Read the model definition and answer for the solid it produces. Units are mm, in the model's axes. A direction names the side the tool comes from. Coordinates: 2 decimals unless noted, no trailing zeros. Write each loop counter-clockwise with the first axis right and the second up, starting at its lowest first coordinate (ties: lowest second). Pieces come first, ordered by that corner, then holes. Notation, with made-up numbers: (80.25, 88.5) -> (138.25, 88.5) arc R19 cw to (138.25, 100.5) -> close; hole circle Ø6 at (42, -27.5). An arc over 180 degrees is marked (long way). Answer as a JSON object with one key per item and string values. Group by question number.
(1) Find section A-A (z = 7.25). Give the vertices of the cut face in (x, y).
(2) Flat-ended cylindrical pins translate along their axes: P1, Ø1.5, axis at x = 4.5, y = 18.5, coming from the -Z side; P2, Ø5.5, axis at y = 10.5, z = 5, coming from the +X side; P3, Ø4, axis at x = 11.5, z = 10, coming from the -Y side. Find the tip coordinate at first contact, or state that the pin passes through.
(3) Find section D-D (y = 5.5). Give the vertices of the cut face in (x, z), then the cut area to 3 significant figures.
(4) Find section B-B (x = 4.1). Give the vertices of the cut face in (y, z).
(5) Straight lines are drawn through the part: L1, parallel to Y at x = 4.1, z = 10.6; L2, parallel to X at y = 19, z = 2.75; L3, parallel to Y at x = 3.5, z = 5.5. For each, find the intervals that lie inside material, in ascending order.
(6) Find section C-C (y = 15.24). Give the vertices of the cut face in (x, z) (3 decimals).
(7) Which of the six approach directions +Z, -Z, +X, -X, +Y, -Y give full straight-line access (tool end or side, diameter ignored) to faces 4 (the face through (6.2, 15.5, 0.8)), 5 (the face through (4, 28.88, 7)), 6 (the face through (10.85, 15.27, 10.61))?
(8) For a pull along Y with two mould halves and no side action, classify faces 1 (the face through (14.034, 15.081, 10.611)), 2 (the face through (10, 15, 9.8)), 3 (the face through (1.6, 15, 5)) as +Y half, -Y half, draft (parallel to the pull), parting line (faces both ways), or undercut.
Autodesk Inventor part; units mm, degrees
ref_plane "YZ Plane" through (0, 0, 0) normal (1, 0, 0) x (0, 1, 0)
ref_plane "XZ Plane" through (0, 0, 0) normal (0, 1, 0) x (-1, 0, 0)
ref_plane "XY Plane" through (0, 0, 0) normal (0, 0, 1) x (1, 0, 0)
sketch "Sketch1" plane through (0, 0, 0) normal (0, 0, 1) x (1, 0, 0)
  line L0 (0, 0) -> (8.2, 0)
  line L1 (8.2, 0) -> (8.2, 30.48)
  line L2 (8.2, 30.48) -> (0, 30.48)
  line L3 (0, 30.48) -> (0, 0)
  line L4 (6.6, 28.88) -> (6.6, 1.6)
  line L5 (6.6, 1.6) -> (1.6, 1.6)
  line L6 (1.6, 1.6) -> (1.6, 28.88)
  line L7 (1.6, 28.88) -> (6.6, 28.88)
  dimension "d0" = 30.48
  dimension "d1" = 8.2
  dimension "d2" = 1.6
extrude "Extrusion1" add sketch "Sketch1" along normal blind 11.4
sketch "Sketch2" plane through (0, 0, 0) normal (0, -1, 0) x (1, 0, 0)
  line L0 (6.6, 0) -> (6.6, 11.4)
  line L1 (1.6, 0) -> (1.6, 11.4)
  line L2 (0, 0) -> (8.2, 0)
  line L3 (1.6, 0) -> (1.6, 2.4)
  line L4 (1.6, 0) -> (1.6, 11.4)
  line L5 (6.6, 0) -> (6.6, 2.4)
  line L6 (6.6, 0) -> (6.6, 11.4)
  line L7 (1.6, 0) -> (6.6, 0)
  arc A0 (6.6, 2.4) -> (1.6, 2.4) centre (4.1, 2.4) ccw
  dimension "d5" = 2.4
  dimension "d6" = 2.4
extrude "Extrusion2" cut sketch "Sketch2" against normal up to surface (30.48 mm away)
sketch "Sketch3" plane through (0, 0, 0) normal (-1, 0, 0) x (0, 0, 1)
  line L0 (0, 30.48) -> (0, 0)
  line L1 (0, 0) -> (11.4, 0)
  line L2 (11.4, 30.48) -> (11.4, 0)
  line L3 (0, 30.48) -> (11.4, 30.48)
  line L4 (0, 0) -> (11.4, 0)
  line L5 (11.4, 30.48) -> (9.8, 30.48)
  line L6 (9.8, 30.48) -> (9.8, 0)
  line L7 (9.8, 0) -> (11.4, 0)
  line L8 (11.4, 0) -> (11.4, 30.48)
  dimension "d9" = 1.6
extrude "Extrusion3" add sketch "Sketch3" against normal up to next contours L3 L2 L1 L6
sketch "Sketch4" plane through (0, 0, 11.4) normal (0, 0, 1) x (1, 0, 0)
  line L0 (0, 0) -> (8.2, 0)
  line L1 (8.2, 0) -> (8.2, 30.48)
  line L2 (8.2, 30.48) -> (0, 30.48)
  line L3 (0, 30.48) -> (0, 0)
  line L4 (6.6, 0) -> (1.6, 0)
  line L5 (4.1, 0) -> (4.1, 30.48)
  line L6 (1.6, 30.48) -> (6.6, 30.48)
  line L7 (8.2, 0) -> (0, 30.48)
  line L8 (8.2, 30.48) -> (0, 0) construction
  circle A0 centre (4.1, 7.84) radius 0.65
  circle A1 centre (4.1, 22.64) radius 0.65
  point P0 (4.1, 15.24)
  dimension "d12" = 7.4
  dimension "d13" = 7.4
  dimension "d14" = 1.3
  dimension "d15" = 1.3
extrude "Extrusion4" cut sketch "Sketch4" against normal up to next contours A0 L5 | L5 A0 | A1 L5 | L5 A1
sketch "Sketch5" plane through (0, 0, 11.4) normal (0, 0, 1) x (1, 0, 0)
  circle A0 centre (4.1, 7.84) radius 0.65
  circle A1 centre (4.1, 22.64) radius 0.65
  line L0 (0, 0) -> (8.2, 0)
  line L1 (8.2, 0) -> (8.2, 30.48)
  line L2 (8.2, 30.48) -> (0, 30.48)
  line L3 (0, 30.48) -> (0, 0)
  line L4 (8.2, 0) -> (0, 30.48)
  line L5 (0, 0) -> (8.2, 30.48)
  circle A2 centre (4.1, 15.24) radius 9.935
  dimension "d18" = 19.87
extrude "Extrusion5" add sketch "Sketch5" against normal blind 1.6 contours A2 L3 | L3 A2 L4 L5 | L5 L4 A2 | A2 L4 L5 L1 | L1 A2 | L4 A2 L5
sketch "Sketch6" plane through (0, 0, 11.4) normal (0, 0, 1) x (1, 0, 0)
  line L0 (1.6, 28.88) -> (1.6, 1.6)
  circle A0 centre (4.1, 22.64) radius 0.65
  circle A1 centre (4.1, 7.84) radius 0.65
  line L1 (0, 6.1905) -> (0, 0)
  line L2 (0, 0) -> (8.2, 0)
  line L3 (8.2, 0) -> (8.2, 6.1905)
  arc A2 (8.2, 6.1905) -> (8.2, 24.2895) centre (4.1, 15.24) ccw
  line L4 (8.2, 24.2895) -> (8.2, 30.48)
  line L5 (8.2, 30.48) -> (0, 30.48)
  line L6 (0, 30.48) -> (0, 24.2895)
  arc A3 (0, 24.2895) -> (0, 6.1905) centre (4.1, 15.24) ccw
  line L7 (8.2, 0) -> (0, 30.48)
  line L8 (8.2, 30.48) -> (0, 0)
  arc A4 (0, 24.2895) -> (0, 6.1905) centre (4.1, 15.24) ccw
  line L9 (-5.835, 15.24) -> (14.035, 15.24) construction
  arc A5 (8.2, 6.1905) -> (8.2, 24.2895) centre (4.1, 15.24) ccw
  circle A6 centre (-3.3, 15.24) radius 0.65
  circle A7 centre (11.5, 15.24) radius 0.65
  dimension "d21" = 7.4
  dimension "d22" = 7.4
  dimension "d23" = 1.3
  dimension "d24" = 1.3
extrude "Extrusion6" cut sketch "Sketch6" against normal up to next contours A6 | A7
sketch "Sketch7" plane through (0, 0, 11.4) normal (0, 0, 1) x (1, 0, 0)
  circle A0 centre (11.5, 15.24) radius 0.65
  circle A1 centre (-3.3, 15.24) radius 0.65
  circle A2 centre (4.1, 22.64) radius 0.65
  circle A3 centre (4.1, 7.84) radius 0.65
  line L0 (0, 6.1905) -> (0, 0)
  line L1 (0, 0) -> (8.2, 0)
  line L2 (8.2, 0) -> (8.2, 6.1905)
  arc A4 (8.2, 6.1905) -> (8.2, 24.2895) centre (4.1, 15.24) ccw
  line L3 (8.2, 24.2895) -> (8.2, 30.48)
  line L4 (8.2, 30.48) -> (0, 30.48)
  line L5 (0, 30.48) -> (0, 24.2895)
  arc A5 (0, 24.2895) -> (0, 6.1905) centre (4.1, 15.24) ccw
  line L6 (0, 0) -> (8.2, 30.48)
  line L7 (0, 30.48) -> (8.2, 0)
  circle A6 centre (4.1, 15.24) radius 1.65
  dimension "d27" = 3.3
extrude "Extrusion7" cut sketch "Sketch7" against normal blind 1.6 contours A6 L7 L6 | L6 L7 A6 | L7 L6 A6 | L7 A6 L6
sketch "Sketch8" plane through (6.6, 30.48, 0) normal (0, 1, 0) x (1, 0, 0)
  line L0 (-5, -2.4) -> (-5, 0)
  line L1 (0, 0) -> (0, -2.4)
  line L2 (-5, -1.2) -> (-3.8, 0)
  line L3 (-5, -1.2) -> (-2.8401, -1.2) construction
  line L4 (-5, 0) -> (-3.8, 0)
  line L5 (0, -1.2) -> (-1.2, 0)
  line L6 (0, 0) -> (-1.2, 0)
  point P0 (-6.6, 0)
  dimension "d30" = 45
extrude "Extrusion8" add sketch "Sketch8" against normal up to surface (30.48 mm away)
fillet "Fillet1" radius 0.2 2 edges at (2.8, 15.24, 0) (5.4, 15.24, 0)
properties part number "CarFrontAxel"
Results below:
{
 "1": {"outline": "(0, 0) -> (8.2, 0) -> (8.2, 30.48) -> (0, 30.48) -> close; hole (1.6, 1.6) -> (6.6, 1.6) -> (6.6, 28.88) -> (1.6, 28.88) -> close"},
 "2": {"P1": "stops at z = 9.8", "P2": "stops at x = 8.2", "P3": "stops at y = 6.9"},
 "3": {"outline": "(0, 0) -> (2.32, 0) arc R0.2 ccw to (2.46, 0.34) -> (1.6, 1.2) -> (1.6, 9.8) -> (6.6, 9.8) -> (6.6, 1.2) -> (5.74, 0.34) arc R0.2 ccw to (5.88, 0) -> (8.2, 0) -> (8.2, 11.4) -> (0, 11.4) -> close", "area": "45.8 mm2"},
 "4": {"outline": "(0, 4.9) -> (1.6, 4.9) -> (1.6, 9.8) -> (7.19, 9.8) -> (7.19, 11.4) -> (0, 11.4) -> close; (8.49, 9.8) -> (13.59, 9.8) -> (13.59, 11.4) -> (8.49, 11.4) -> close; (16.89, 9.8) -> (21.99, 9.8) -> (21.99, 11.4) -> (16.89, 11.4) -> close; (23.29, 9.8) -> (28.88, 9.8) -> (28.88, 4.9) -> (30.48, 4.9) -> (30.48, 11.4) -> (23.29, 11.4) -> close"},
 "5": {"L1": "y = 0 to 7.19, 8.49 to 13.59, 16.89 to 21.99, 23.29 to 30.48", "L2": "x = 0 to 1.6, 6.6 to 8.2", "L3": "y = 0 to 1.6, 28.88 to 30.48"},
 "6": {"outline": "(-5.835, 9.8) -> (-3.95, 9.8) -> (-3.95, 11.4) -> (-5.835, 11.4) -> close; (-2.65, 9.8) -> (0, 9.8) -> (0, 0) -> (2.317, 0) arc R0.2 ccw to (2.459, 0.341) -> (1.6, 1.2) -> (1.6, 9.8) -> (2.45, 9.8) -> (2.45, 11.4) -> (-2.65, 11.4) -> close; (5.741, 0.341) arc R0.2 ccw to (5.883, 0) -> (8.2, 0) -> (8.2, 9.8) -> (10.85, 9.8) -> (10.85, 11.4) -> (5.75, 11.4) -> (5.75, 9.8) -> (6.6, 9.8) -> (6.6, 1.2) -> close; (12.15, 9.8) -> (14.035, 9.8) -> (14.035, 11.4) -> (12.15, 11.4) -> close"},
 "7": {"face 4": "+Y, -Y", "face 5": "none", "face 6": "+Z, -Z"},
 "8": {"face 1": "parting line", "face 2": "draft", "face 3": "undercut"}
}
